from build123d import *

# Parameters (mm, degrees)
BOSS_EXTRUDE2_DEPTH = 3
CUT_EXTRUDE1_REACH  = 58.648
SKETCH3_R           = 1.5
SKETCH4_R           = 15.5
SKETCH4_R_2         = 1.5
CUT_EXTRUDE2_DEPTH  = 3


with BuildPart() as part:
    # Sketch2 → Boss-Extrude2 (new body)
    with BuildSketch(Plane.XY):
        with BuildLine():
            Line((-10, -29.342801502), (-10, -38.729833462))
            ThreePointArc((-10, -38.729833462), (0, -40), (10, -38.729833462))
            Line((10, -38.729833462), (10, -29.342801502))
            ThreePointArc((10, -29.342801502), (21.920310217, -21.920310217), (29.342801502, -10))
            Line((29.342801502, -10), (38.729833462, -10))
            ThreePointArc((38.729833462, -10), (40, 0), (38.729833462, 10))
            Line((38.729833462, 10), (29.342801502, 10))
            ThreePointArc((29.342801502, 10), (21.920310217, 21.920310217), (10, 29.342801502))
            Line((10, 29.342801502), (10, 38.729833462))
            ThreePointArc((10, 38.729833462), (0, 40), (-10, 38.729833462))
            Line((-10, 38.729833462), (-10, 29.342801502))
            ThreePointArc((-10, 29.342801502), (-21.920310217, 21.920310217), (-29.342801502, 10))
            Line((-29.342801502, 10), (-38.729833462, 10))
            ThreePointArc((-38.729833462, 10), (-40, 0), (-38.729833462, -10))
            Line((-38.729833462, -10), (-29.342801502, -10))
            ThreePointArc((-29.342801502, -10), (-21.920310217, -21.920310217), (-10, -29.342801502))
        make_face()
    extrude(amount=BOSS_EXTRUDE2_DEPTH)

    # Sketch3 → Cut-Extrude1 (cut, up to next)
    with BuildSketch(Plane.XY.offset(3), mode=Mode.PRIVATE) as cut_extrude1_sk1:
        with Locations((0, 35)):
            Circle(SKETCH3_R)
    cut_extrude1_tool1 = extrude(cut_extrude1_sk1.sketch, amount=-CUT_EXTRUDE1_REACH, mode=Mode.PRIVATE) & part.part
    # Sketch3 → Cut-Extrude1 (cut, up to next)
    with BuildSketch(Plane.XY.offset(3), mode=Mode.PRIVATE) as cut_extrude1_sk2:
        with Locations((35, 0)):
            Circle(SKETCH3_R)
    cut_extrude1_tool2 = extrude(cut_extrude1_sk2.sketch, amount=-CUT_EXTRUDE1_REACH, mode=Mode.PRIVATE) & part.part
    # Sketch3 → Cut-Extrude1 (cut, up to next)
    with BuildSketch(Plane.XY.offset(3), mode=Mode.PRIVATE) as cut_extrude1_sk3:
        with Locations((0, -35)):
            Circle(SKETCH3_R)
    cut_extrude1_tool3 = extrude(cut_extrude1_sk3.sketch, amount=-CUT_EXTRUDE1_REACH, mode=Mode.PRIVATE) & part.part
    # Sketch3 → Cut-Extrude1 (cut, up to next)
    with BuildSketch(Plane.XY.offset(3), mode=Mode.PRIVATE) as cut_extrude1_sk4:
        with Locations((-35, 0)):
            Circle(SKETCH3_R)
    cut_extrude1_tool4 = extrude(cut_extrude1_sk4.sketch, amount=-CUT_EXTRUDE1_REACH, mode=Mode.PRIVATE) & part.part
    add(cut_extrude1_tool1.solids().sort_by_distance((0, 35, 3))[0], mode=Mode.SUBTRACT)
    add(cut_extrude1_tool2.solids().sort_by_distance((35, 0, 3))[0], mode=Mode.SUBTRACT)
    add(cut_extrude1_tool3.solids().sort_by_distance((0, -35, 3))[0], mode=Mode.SUBTRACT)
    add(cut_extrude1_tool4.solids().sort_by_distance((-35, 0, 3))[0], mode=Mode.SUBTRACT)

    # Sketch4 → Cut-Extrude2 (cut)
    with BuildSketch(Plane.XY.offset(3)):
        Circle(SKETCH4_R)
        with Locations((-13, 13)):
            Circle(SKETCH4_R_2)
        with Locations(Location((-13, -13, 0), (0, 0, 180))):
            Circle(SKETCH4_R_2)
        with Locations((13, -13)):
            Circle(SKETCH4_R_2)
        with Locations(Location((13, 13, 0), (0, 0, 180))):
            Circle(SKETCH4_R_2)
    extrude(amount=-CUT_EXTRUDE2_DEPTH, mode=Mode.SUBTRACT)


solid = part.part
Source: CAD feature listing. Evaluate the final solid. Frame: model axes, mm. A direction names the side the tool comes from. Give positions to 0.01 mm unless a question says otherwise; leave off trailing zeros. Write each loop counter-clockwise with the first axis right and the second up, starting at its lowest first coordinate (ties: lowest second). Pieces come first, ordered by that corner, then holes. Notation, with made-up numbers: (-23.75, 43) -> (-5.75, 43) arc R21 cw to (-5.75, 61) -> close; hole circle Ø8 at (13, -32.75). An arc over 180 degrees is marked (long way). Return JSON: item names as keys, results as strings. Group by question number.
1. Access query for faces 1 (the face through (-34, 10, 1)), 2 (the face through (34, 10, 1)), 3 (the face through (-22.06, -21.78, 1.48)), 4 (the face through (-2.018, 15.368, 1.521)), 5 (the face through (34, -10, 1)). Directions: +Z, -Z, +X, -X, +Y, -Y. A direction counts if a zero-diameter tool reaches every point of the face in a straight line with its end or side. Return the directions, or none.
2. Material intervals for line 1 (Y direction, x = 0, z = 1.15); line 2 (X direction, y = 32, z = 2.05); line 3 (X direction, y = -2.5, z = 1.25), sorted ascending. Write a range as from..to.
3. Section B-B, the plane x = 0. Output: boundary loops of the cut face in (y, z), then the cut area to 3 significant figures.
4. Mould query, pull axis Y, two halves, no side actions, for faces 6 (the face through (-0.325, 33.536, 1.521)), 7 (the face through (10, -34, 1)), 8 (the face through (0, -40, 1)). Classes: +Y half, -Y half, draft (parallel to the pull), parting line (faces both ways), or undercut.
5. Pin query (flat end, axial travel): pin 1 Ø1 at (y, z) = (-25.5, 1.5) entering from -X; pin 2 Ø0.9 at (y, z) = (-33, 1) entering from +X; pin 3 Ø0.9 at (x, z) = (33.5, 1) entering from +Y. Return the tip coordinate at first contact, or that it passes through.
6. Section C-C, the plane z = 1.75. Count the separate pieces of the cut face and the enclosed holes in it, then the cut area to 3 significant figures.
7. Section A-A, the plane y = 35. Output: boundary loops of the cut face in (x, z), then the cut area to 3 significant figures.
Determined:
{
 "1": {"face 1": "+Z, -Z, -X, +Y", "face 2": "+Z, -Z, +X, +Y", "face 3": "+Z, -Z, -X, -Y", "face 4": "+Z, -Z", "face 5": "+Z, -Z, +X, -Y"},
 "2": {"line 1": "y = -40..-36.5, -33.5..-15.5, 15.5..33.5, 36.5..40", "line 2": "x = -10..10", "line 3": "x = -39.92..-15.3, 15.3..39.92"},
 "3": {"outline": "(-40, 0) -> (-36.5, 0) -> (-36.5, 3) -> (-40, 3) -> close; (-33.5, 0) -> (-15.5, 0) -> (-15.5, 3) -> (-33.5, 3) -> close; (15.5, 0) -> (33.5, 0) -> (33.5, 3) -> (15.5, 3) -> close; (36.5, 0) -> (40, 0) -> (40, 3) -> (36.5, 3) -> close", "area": "129 mm2"},
 "4": {"face 6": "undercut", "face 7": "draft", "face 8": "-Y half"},
 "5": {"pin 1": "stops at x = -18.33", "pin 2": "stops at x = 10", "pin 3": "stops at y = 10"},
 "6": {"separate pieces": "1", "enclosed holes": "9", "area": "2,940 mm2"},
 "7": {"outline": "(-10, 0) -> (-1.5, 0) -> (-1.5, 3) -> (-10, 3) -> close; (1.5, 0) -> (10, 0) -> (10, 3) -> (1.5, 3) -> close", "area": "51.0 mm2"}
}
